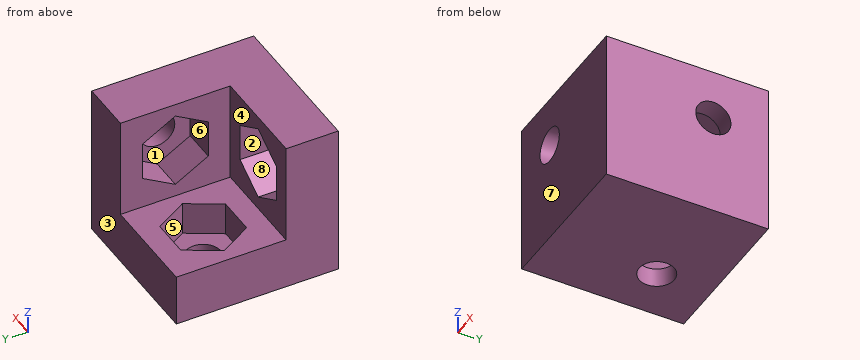
from build123d import *

# Parameters (mm, degrees)
F1_DEPTH  = 10
F2_R      = 1.6
F3_DEPTH  = 3
F4_DEPTH  = 25
F5_R      = 1.6
F6_DEPTH  = 3
F7_DEPTH  = 25
F8_W      = 9.25
F8_H      = 9.25
F9_DEPTH  = 4.75
F10_R     = 1.6
F11_DEPTH = 3
F12_DEPTH = 25


with BuildPart() as f1:
    # F0 (on Front) → F1 (new body)
    with BuildSketch(Plane.XZ):
        Polygon((-14, 0), (0, 0), (0, 14), (-4.75, 14), (-4.75, 4.75), (-14, 4.75), align=None)
    extrude(amount=F1_DEPTH)

    # F2 (on face) → F3 (cut)
    with BuildSketch(Plane(origin=(-4.75, 0, 0), x_dir=(0, -1, 0), z_dir=(-1, 0, 0))):
        Polygon((2, 11.1070508076), (2, 7.6429491924), (5, 5.9108983849), (8, 7.6429491924), (8, 11.1070508076), (5, 12.8391016151), align=None)
        with Locations((5, 9.375)):
            Circle(F2_R, mode=Mode.SUBTRACT)
    extrude(amount=-F3_DEPTH, mode=Mode.SUBTRACT)

    # F4 (cut): a face of the model
    f4_faces = [f1.faces().sort_by_distance(p)[0] for p in [
        (-4.75, -5, 9.375),
    ]]
    extrude(f4_faces, amount=-F4_DEPTH, mode=Mode.SUBTRACT)

    # F5 (on face) → F6 (cut)
    with BuildSketch(Plane.XY.offset(4.75)):
        Polygon((-11.1070508076, -8), (-7.6429491924, -8), (-5.9108983849, -5), (-7.6429491924, -2), (-11.1070508076, -2), (-12.8391016151, -5), align=None)
        with Locations((-9.375, -5)):
            Circle(F5_R, mode=Mode.SUBTRACT)
    extrude(amount=-F6_DEPTH, mode=Mode.SUBTRACT)

    # F7 (cut): a face of the model
    f7_faces = [f1.faces().sort_by_distance(p)[0] for p in [
        (-9.375, -5, 4.75),
    ]]
    extrude(f7_faces, amount=-F7_DEPTH, mode=Mode.SUBTRACT)

    # F8 (on face) → F9 (join)
    with BuildSketch(Plane.XZ.offset(10)):
        with Locations((-9.375, 9.375)):
            Rectangle(F8_W, F8_H)
        Polygon((-14, 0), (0, 0), (0, 14), (-4.75, 14), (-4.75, 4.75), (-14, 4.75), align=None)
    extrude(amount=F9_DEPTH)

    # F10 (on face) → F11 (cut)
    with BuildSketch(Plane(origin=(0, -10, 0), x_dir=(-1, 0, 0), z_dir=(0, 1, 0))):
        Polygon((6.375, 11.1070508076), (6.375, 7.6429491924), (9.375, 5.9108983849), (12.375, 7.6429491924), (12.375, 11.1070508076), (9.375, 12.8391016151), align=None)
        with Locations((9.375, 9.375)):
            Circle(F10_R, mode=Mode.SUBTRACT)
    extrude(amount=-F11_DEPTH, mode=Mode.SUBTRACT)

    # F12 (cut): a face of the model
    f12_faces = [f1.faces().sort_by_distance(p)[0] for p in [
        (-9.375, -10, 9.375),
    ]]
    extrude(f12_faces, amount=-F12_DEPTH, mode=Mode.SUBTRACT)


solid = f1.part
Verification items for the finished model (mm, model axes). Face numbers are marked on the shaded views. A direction names the side the tool comes from. Coordinates: 2 decimals unless noted, no trailing zeros. Order: outer loops, then holes, each group sorted by start corner. A loop starts at its lowest first (then second) coordinate and runs counter-clockwise, first axis right, second up. Notation, with made-up numbers: M 31,-27.75 L 79,-27.75 A6 cw 79,-23.75 Z; hole C -23.75,75 d1. An arc over 180 degrees is marked long. One line per item, written item: value. Start each with the question number.
Item 1: Sectioned sample at C-C (y = -7.25). Enter the section's corners in (x, z).
Item 2: Sectioned sample at D-D (z = 11.75). Enter the section's corners in (x, y).
Item 3: Sectioned sample at A-A (x = -3.5). Enter the section's corners in (y, z), then the cut area to 3 significant figures.
Item 4: Access from +Z, -Z, +X, -X, +Y, -Y to the whole of each face (thin tool, end or side, straight path). Record for the marked faces 4, 5, 6, 7 and 8.
Item 5: Mould release check, pull along X, two halves, no side actions. Record for the marked faces 1, 2 and 3: released by +X, released by -X, zero draft, split by the parting line, or undercut.
Item 6: Scan lines: probe 1 along Y at (x, z) = (-5, 6.75); probe 2 along Z at (x, y) = (-1.3, -5) (3 decimals); probe 3 along Z at (x, y) = (-9.75, -2.5). Record each from-to range of solid material in increasing order.
Item 7: Sectioned sample at B-B (z = 2). Enter the section's corners in (x, y).
Item 8: Gauge pin test, flat ends, axial feed: pin 1 (3 mm diameter, centred on x = -9.5, y = -4.5, fed in from +Z); pin 2 (1.5 mm diameter, centred on y = -8, z = 9.5, fed in from -X); pin 3 (1 mm diameter, centred on x = -12.5, z = 12.5, fed in from +Y). Record the tip position at first contact, or that the pin passes through.
Conclusion:
1. outline: M -14,0 L 0,0 L 0,14 L -4.75,14 L -4.75,11.54 L -1.75,11.54 L -1.75,7.21 L -4.75,7.21 L -4.75,4.75 L -7.21,4.75 L -7.21,1.75 L -11.54,1.75 L -11.54,4.75 L -14,4.75 Z
2. outline: M -14,-14.75 L 0,-14.75 L 0,0 L -4.75,0 L -4.75,-3.11 L -1.75,-3.11 L -1.75,-6.89 L -4.75,-6.89 L -4.75,-10 L -7.49,-10 L -7.49,-13 L -11.26,-13 L -11.26,-10 L -14,-10 Z
3. outline: M -14.75,0 L 0,0 L 0,14 L -14.75,14 Z; hole M -8,7.64 L -5,5.91 L -2,7.64 L -2,11.11 L -5,12.84 L -8,11.11 Z
3. area: 175 mm^2
4. face 4: +Z, -X, +Y
4. face 5: +Z
4. face 6: -X
4. face 7: +Z, -Z, +X, -X, -Y
4. face 8: +Y
5. face 1: released by -X
5. face 2: undercut
5. face 3: zero draft
6. probe 1: y = -14.75 to -10
6. probe 2: z = 0 to 7.775, 10.975 to 14
6. probe 3: z = 0 to 1.75
7. outline: M -14,-14.75 L 0,-14.75 L 0,0 L -14,0 Z; hole M -12.84,-5 L -11.11,-8 L -7.64,-8 L -5.91,-5 L -7.64,-2 L -11.11,-2 Z
8. pin 1: stops at z = 1.75
8. pin 2: stops at x = -4.75
8. pin 3: stops at y = -10
